from build123d import *

# Parameters (mm, degrees)
CROQUIS1_R              = 1.45
SALIENTE_EXTRUIR1_DEPTH = 6
REDONDEO1_R             = 0.5
REDONDEO2_R             = 8


with BuildPart() as part:
    # Croquis1 → Saliente-Extruir1 (new body)
    with BuildSketch(Plane(origin=(0, 0, 0), x_dir=(1, 0, 0), z_dir=(0, 1, 0))):
        with BuildLine():
            Line((24.75319, -28.652334501), (27.25319, -26.502334501))
            Line((27.25319, -26.502334501), (27.25319, -22.652334501))
            Line((27.25319, -22.652334501), (27.25319, -21.152334501))
            Line((27.25319, -21.152334501), (26.25319, -21.152334501))
            Line((26.25319, -21.152334501), (25.90319, -21.652334501))
            Line((25.90319, -21.652334501), (25.55319, -21.152334501))
            Line((25.55319, -21.152334501), (25.35319, -21.152334501))
            Line((25.35319, -21.152334501), (25.00319, -21.652334501))
            Line((25.00319, -21.652334501), (24.65319, -21.152334501))
            Line((24.65319, -21.152334501), (24.45319, -21.152334501))
            Line((24.45319, -21.152334501), (24.10319, -21.652334501))
            Line((24.10319, -21.652334501), (23.75319, -21.152334501))
            Line((23.75319, -21.152334501), (23.55319, -21.152334501))
            Line((23.55319, -21.152334501), (23.20319, -21.652334501))
            Line((23.20319, -21.652334501), (22.85319, -21.152334501))
            Line((22.85319, -21.152334501), (22.65319, -21.152334501))
            Line((22.65319, -21.152334501), (22.30319, -21.652334501))
            Line((22.30319, -21.652334501), (21.95319, -21.152334501))
            Line((21.95319, -21.152334501), (21.75319, -21.152334501))
            Line((21.75319, -21.152334501), (21.40319, -21.652334501))
            Line((21.40319, -21.652334501), (21.05319, -21.152334501))
            Line((21.05319, -21.152334501), (20.85319, -21.152334501))
            Line((20.85319, -21.152334501), (20.50319, -21.652334501))
            Line((20.50319, -21.652334501), (20.15319, -21.152334501))
            Line((20.15319, -21.152334501), (19.95319, -21.152334501))
            Line((19.95319, -21.152334501), (19.60319, -21.652334501))
            Line((19.60319, -21.652334501), (19.25319, -21.152334501))
            Line((19.25319, -21.152334501), (19.05319, -21.152334501))
            Line((19.05319, -21.152334501), (18.70319, -21.652334501))
            Line((18.70319, -21.652334501), (18.35319, -21.152334501))
            Line((18.35319, -21.152334501), (18.15319, -21.152334501))
            Line((18.15319, -21.152334501), (17.80319, -21.652334501))
            Line((17.80319, -21.652334501), (17.45319, -21.152334501))
            Line((17.45319, -21.152334501), (17.25319, -21.152334501))
            Line((17.25319, -21.152334501), (16.90319, -21.652334501))
            Line((16.90319, -21.652334501), (16.55319, -21.152334501))
            Line((16.55319, -21.152334501), (16.35319, -21.152334501))
            Line((16.35319, -21.152334501), (16.00319, -21.652334501))
            Line((16.00319, -21.652334501), (15.65319, -21.152334501))
            Line((15.65319, -21.152334501), (15.45319, -21.152334501))
            Line((15.45319, -21.152334501), (15.10319, -21.652334501))
            Line((15.10319, -21.652334501), (14.75319, -21.152334501))
            Line((14.75319, -21.152334501), (14.55319, -21.152334501))
            Line((14.55319, -21.152334501), (14.20319, -21.652334501))
            Line((14.20319, -21.652334501), (13.85319, -21.152334501))
            Line((13.85319, -21.152334501), (13.65319, -21.152334501))
            Line((13.65319, -21.152334501), (13.30319, -21.652334501))
            Line((13.30319, -21.652334501), (12.95319, -21.152334501))
            Line((12.95319, -21.152334501), (12.75319, -21.152334501))
            Line((12.75319, -21.152334501), (12.40319, -21.652334501))
            Line((12.40319, -21.652334501), (12.05319, -21.152334501))
            Line((12.05319, -21.152334501), (11.85319, -21.152334501))
            Line((11.85319, -21.152334501), (11.50319, -21.652334501))
            Line((11.50319, -21.652334501), (11.15319, -21.152334501))
            Line((11.15319, -21.152334501), (10.95319, -21.152334501))
            Line((10.95319, -21.152334501), (10.60319, -21.652334501))
            Line((10.60319, -21.652334501), (10.25319, -21.152334501))
            Line((10.25319, -21.152334501), (10.05319, -21.152334501))
            Line((10.05319, -21.152334501), (9.70319, -21.652334501))
            Line((9.70319, -21.652334501), (9.35319, -21.152334501))
            Line((9.35319, -21.152334501), (9.15319, -21.152334501))
            Line((9.15319, -21.152334501), (8.80319, -21.652334501))
            Line((8.80319, -21.652334501), (8.45319, -21.152334501))
            Line((8.45319, -21.152334501), (8.25319, -21.152334501))
            Line((8.25319, -21.152334501), (7.90319, -21.652334501))
            Line((7.90319, -21.652334501), (7.55319, -21.152334501))
            Line((7.55319, -21.152334501), (7.35319, -21.152334501))
            Line((7.35319, -21.152334501), (7.25319, -21.152334501))
            Line((7.25319, -21.152334501), (5.49119, -22.652334501))
            Line((5.49119, -22.652334501), (-5.24681, -22.652334501))
            Line((-5.24681, -22.652334501), (-8.231533319, -22.652334501))
            Line((-8.231533319, -22.652334501), (-24.994112506, -30.755671031))
            ThreePointArc((-24.994112506, -30.755671031), (-26.854466, -36.097869537), (-21.512267494, -37.958223031))
            Line((-21.512267494, -37.958223031), (-2.262086681, -28.652334501))
            Line((-2.262086681, -28.652334501), (24.75319, -28.652334501))
        make_face()
        with Locations(Location((21.75319, -24.902334501, 0), (0, 0, 270))):
            Circle(CROQUIS1_R, mode=Mode.SUBTRACT)
        with Locations(Location((-5.24681, -25.652334501, 0), (0, 0, 270))):
            Circle(CROQUIS1_R, mode=Mode.SUBTRACT)
        with Locations(Location((-23.25319, -34.356947031, 0), (0, 0, 270))):
            Circle(CROQUIS1_R, mode=Mode.SUBTRACT)
    extrude(amount=SALIENTE_EXTRUIR1_DEPTH)

    # Redondeo1
    redondeo1_edges = [part.edges().sort_by_distance(p)[0] for p in [
        (27.25319, 3, 21.152334501),
        (27.25319, 3, 26.502334501),
        (24.75319, 3, 28.652334501),
    ]]
    fillet(redondeo1_edges, radius=REDONDEO1_R)

    # Redondeo2
    redondeo2_edges = [part.edges().sort_by_distance(p)[0] for p in [
        (-8.231533319, 3, 22.652334501),
        (-2.262086681, 3, 28.652334501),
    ]]
    fillet(redondeo2_edges, radius=REDONDEO2_R)


solid = part.part
Read the model definition and answer for the solid it produces. Units are mm, in the model's axes. A direction names the side the tool comes from. Coordinates: 2 decimals unless noted, no trailing zeros. Loops run counter-clockwise (first coordinate to the right, second up) from the corner with the lowest first, then second, coordinate; pieces in that order, holes last.
Q1. The part is cut by section A-A on x = 4. Write down the section's boundary in (y, z).
Q2. Each of these flat-tipped pins is pushed along its axis until it touches: pin 1 Ø2 at (x, y) = (-12.5, 0.5) entering from +Z; pin 2 Ø1.5 at (y, z) = (5, 28.5) entering from +X; pin 3 Ø2 at (y, z) = (5, 29.5) entering from +X. Where does it stop, or does it pass through?
Q3. Consider probe 1 along X at (y, z) = (2.75, 33.75); probe 2 along Z at (x, y) = (-24, 5.7); probe 3 along Z at (x, y) = (23, 1.15). Determine where each line is inside the solid, lowest interval first.
Q4. Which of the six approach directions +Z, -Z, +X, -X, +Y, -Y give full straight-line access (tool end or side, diameter ignored) to faces 4 (the face through (12, 3, 28.652)), 5 (the face through (0, 3, 22.652)), 6 (the face through (-4.27, 2.96, 24.58))?
Q5. The mould has two halves that part along X. Classify faces 1 (the face through (-26.9, 3, 36)), 2 (the face through (-22.82, 2.96, 35.74)), 3 (the face through (0, 6, 28)): +X half, -X half, draft (parallel to the pull), parting line (faces both ways), or undercut.
Q6. The part is cut by section B-B on z = 31.75. Write down the section's boundary in (x, y).
Q7. The part is cut by section C-C on y = 2.8. Give the number of separate pieces and of enclosed holes in the cut face, and give its area (3 significant figures).
Results below:
1. outline: (0, 22.65) - (6, 22.65) - (6, 28.65) - (0, 28.65) - close
2. pin 1: stops at z = 34.08
2. pin 2: stops at x = 25.8
2. pin 3: stops at x = 24.93
3. probe 1: x = -27.21 to -24.57, -21.94 to -12.81
3. probe 2: z = 30.28 to 33.11, 35.6 to 38.29
3. probe 3: z = 21.36 to 24.16, 25.64 to 28.65
4. face 4: +Z, +X, +Y, -Y
4. face 5: -Z, -X, +Y, -Y
4. face 6: +Y, -Y
5. face 1: parting line
5. face 2: undercut
5. face 3: draft
6. outline: (-26.29, 0) - (-8.67, 0) - (-8.67, 6) - (-26.29, 6) - close
7. separate pieces: 1
7. enclosed holes: 3
7. area: 385 mm2
